from build123d import *

# Parameters (mm, degrees)
SKETCH1_W                                       = 100
SKETCH1_H                                       = 60
BOSS_EXTRUDE1_DEPTH                             = 50
CBORE_FOR_M5_HEX_HEAD_BOLT1_D                   = 14
CBORE_FOR_M5_HEX_HEAD_BOLT1_DEPTH               = 16
CBORE_FOR_M5_HEX_HEAD_BOLT1_CBORE_D             = 20
CBORE_FOR_M5_HEX_HEAD_BOLT1_CBORE_DEPTH         = 3
CBORE_FOR_M5_HEX_HEAD_BOLT1_TIP                 = 4.206024333
CSK_FOR_M5_FLAT_HEAD_MACHINE_SCREW1_D           = 16
CSK_FOR_M5_FLAT_HEAD_MACHINE_SCREW1_DEPTH       = 16
CSK_FOR_M5_FLAT_HEAD_MACHINE_SCREW1_CSINK_D     = 24
CSK_FOR_M5_FLAT_HEAD_MACHINE_SCREW1_CSINK_ANGLE = 90
CSK_FOR_M5_FLAT_HEAD_MACHINE_SCREW1_TIP         = 4.806884952
M16X2_0_TAPPED_HOLE1_D                          = 14


with BuildPart() as part:
    # Sketch1 → Boss-Extrude1 (new body)
    with BuildSketch(Plane(origin=(0, 0, 0), x_dir=(1, 0, 0), z_dir=(0, 1, 0))):
        with Locations((50, 30)):
            Rectangle(SKETCH1_W, SKETCH1_H)
    extrude(amount=-BOSS_EXTRUDE1_DEPTH)

    # CBORE for M5 Hex Head Bolt1
    with Locations(Plane(origin=(0, 0, 0), x_dir=(1, 0, 0), z_dir=(0, 1, 0))):
        with Locations((50, 30)):
            CounterBoreHole(CBORE_FOR_M5_HEX_HEAD_BOLT1_D / 2, CBORE_FOR_M5_HEX_HEAD_BOLT1_CBORE_D / 2, CBORE_FOR_M5_HEX_HEAD_BOLT1_CBORE_DEPTH, depth=CBORE_FOR_M5_HEX_HEAD_BOLT1_DEPTH)
            with Locations((0, 0, -(CBORE_FOR_M5_HEX_HEAD_BOLT1_DEPTH + CBORE_FOR_M5_HEX_HEAD_BOLT1_TIP / 2))):  # 118° drill point
                Cone(0, CBORE_FOR_M5_HEX_HEAD_BOLT1_D / 2, CBORE_FOR_M5_HEX_HEAD_BOLT1_TIP, mode=Mode.SUBTRACT)

    # CSK for M5 Flat Head Machine Screw1
    with Locations(Plane(origin=(0, 0, 0), x_dir=(1, 0, 0), z_dir=(0, 1, 0))):
        with Locations((80, 30)):
            CounterSinkHole(CSK_FOR_M5_FLAT_HEAD_MACHINE_SCREW1_D / 2, CSK_FOR_M5_FLAT_HEAD_MACHINE_SCREW1_CSINK_D / 2, depth=CSK_FOR_M5_FLAT_HEAD_MACHINE_SCREW1_DEPTH, counter_sink_angle=CSK_FOR_M5_FLAT_HEAD_MACHINE_SCREW1_CSINK_ANGLE)
            with Locations((0, 0, -(CSK_FOR_M5_FLAT_HEAD_MACHINE_SCREW1_DEPTH + CSK_FOR_M5_FLAT_HEAD_MACHINE_SCREW1_TIP / 2))):  # 118° drill point
                Cone(0, CSK_FOR_M5_FLAT_HEAD_MACHINE_SCREW1_D / 2, CSK_FOR_M5_FLAT_HEAD_MACHINE_SCREW1_TIP, mode=Mode.SUBTRACT)

    # M16x2.0 Tapped Hole1 (through all)
    with Locations(Plane(origin=(0, 0, 0), x_dir=(1, 0, 0), z_dir=(0, 1, 0))):
        with Locations((20, 30)):
            Hole(M16X2_0_TAPPED_HOLE1_D / 2)


solid = part.part
Part model, mm, in its own coordinate system. A direction names the side the tool comes from. Coordinates: 2 decimals unless noted, no trailing zeros. Loops run counter-clockwise (first coordinate to the right, second up) from the corner with the lowest first, then second, coordinate; pieces in that order, holes last. Notation, with made-up numbers: M -24,-4 L 9,-4 A18 ccw 9,6 Z; hole C 39,-6 d6. An arc over 180 degrees is marked long. Use a Markdown table: item, result. Add a question column.
Q1. Pin check, flat tips, straight feed: P1, Ø8, axis at y = -24.5, z = -20.5, coming from the -X side; P2, Ø16, axis at x = 50, z = -30, coming from the +Y side. Stop position of each tip, or through.
Q2. Mould opens along X. For faces 1 (the cylindrical face through (85.9, -10.1, -35.4)), 2 (the flat face through (100, -25, -30)), 3 (the flat face through (38, 0, -30)), 4 (the conical face through (51.16, -19.476, -30.365)) say: +X half, -X half, draft (parallel to the pull), parting line (faces both ways), or undercut.
Q3. Cut at A-A (x = 20). Write the cut outline in (y, z).
Q4. Cut at B-B (y = -14.5). Write the cut outline in (x, z), and give its area (3 significant figures).
Q5. Cut at C-C (y = -43.5). Write the cut outline in (x, z), and give its area (3 significant figures).
Q6. Which spindle directions (+Z, -Z, +X, -X, +Y, -Y) get a long thin tool onto all of the face, cutting with end or side? Do faces 5 (the flat face through (49, -50, -30)), 6 (the flat face through (43, -3, -28)). Say none if no direction does.
Q7. Probe L1, parallel to X at y = -39, z = -30; L2, parallel to Z at x = 20, y = -36.5; L3, parallel to Y at x = 71.5, z = -26.5. List the from-to ranges inside material, lowest first.
Worked out:
| question | item | result |
|---|---|---|
| 1 | P1 | stops at x = 0 |
| 1 | P2 | stops at y = -3 |
| 2 | face 1 | undercut |
| 2 | face 2 | +X half |
| 2 | face 3 | draft |
| 2 | face 4 | undercut |
| 3 | outline | M -50,-60 L 0,-60 L 0,-37 L -50,-37 Z; M -50,-23 L 0,-23 L 0,0 L -50,0 Z |
| 4 | outline | M 0,-60 L 100,-60 L 100,0 L 0,0 Z; hole C 20,-30 d14; hole C 50,-30 d14; hole C 80,-30 d16 |
| 4 | area | 5,490 mm2 |
| 5 | outline | M 0,-60 L 100,-60 L 100,0 L 0,0 Z; hole C 20,-30 d14 |
| 5 | area | 5,850 mm2 |
| 6 | face 5 | +Z, -Z, +X, -X, -Y |
| 6 | face 6 | +Y |
| 7 | L1 | x = 0 to 13, 27 to 100 |
| 7 | L2 | z = -60 to -37, -23 to 0 |
| 7 | L3 | y = -50 to -2.81 |
